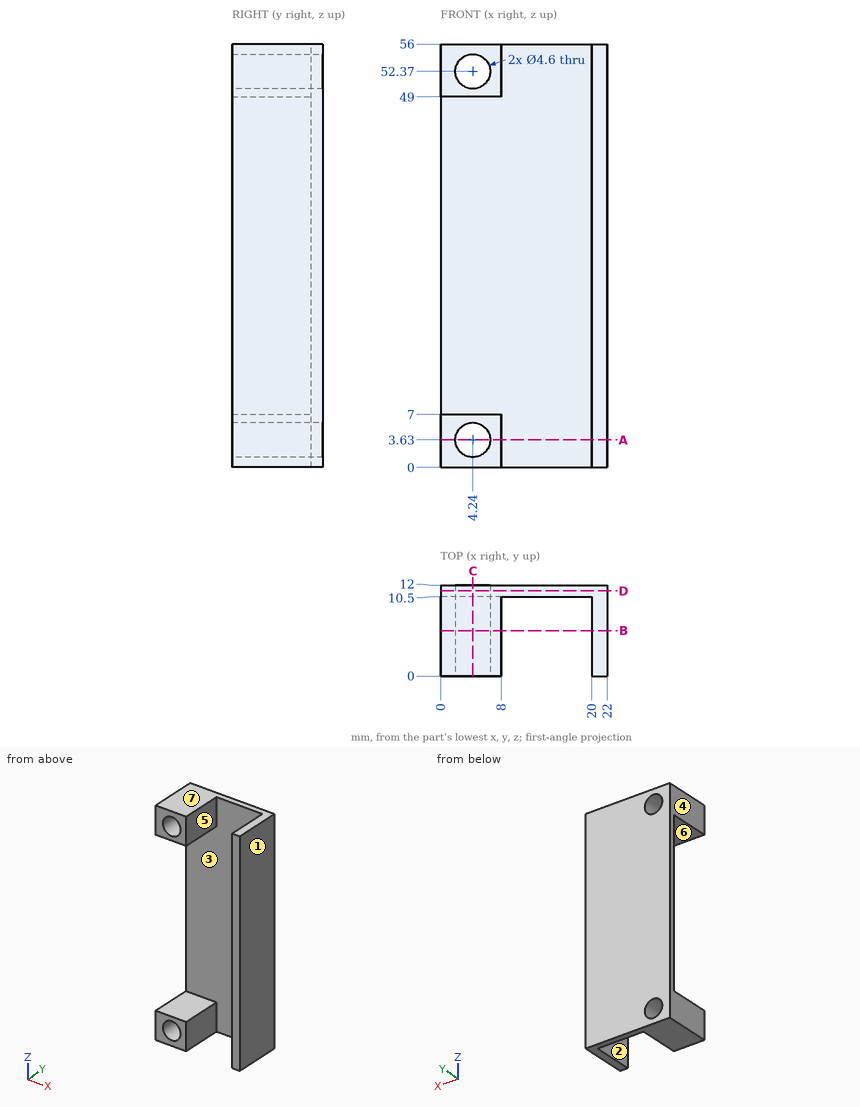
Geometry check sheet. Reference: drawing and pictorial views, mm from the part's lowest x, y, z. A direction names the side the tool comes from. Round coordinates to 2 decimals unless told otherwise and drop trailing zeros. Write each loop counter-clockwise with the first axis right and the second up, starting at its lowest first coordinate (ties: lowest second). Pieces come first, ordered by that corner, then holes. Notation, with made-up numbers: (19, -17) -> (47, -17) arc R25 cw to (47, -2) -> close; hole circle Ø5 at (23, 50.25). An arc over 180 degrees is marked (long way). Answer as CSV lines item,"result". Start each with the question number.
1) Section check C-C on x = 4.24. Enter the section's corners in (y, z), and give its area (3 significant figures).
2) Tool access check on the marked faces 5, 6 and 7. Record the directions out of +Z, -Z, +X, -X, +Y, -Y that give a thin tool (end or side, any length) a straight path to the whole face; none if there is none.
3) Section check D-D on y = 11.25. Enter the section's corners in (x, z), and give its area (3 significant figures).
4) Section check A-A on z = 3.63. Enter the section's corners in (x, y), and give its area (3 significant figures).
5) Section check B-B on y = 6. Enter the section's corners in (x, z), and give its area (3 significant figures).
6) Release check for a two-part mould opening along X. For the marked faces 1, 2, 3 and 4 record: pulls with the +X half, pulls with the -X half, needs draft (parallel to the pull), parting line crosses it, or undercut.
7) Material ranges on line 1 (X direction, y = 8.25, z = 52.37); line 2 (X direction, y = 7.5, z = 50); line 3 (Y direction, x = 17.75, z = 11), recorded low to high. Write a range as from..to.
8) Go/stop test with flat-tipped pins: P1, Ø3, axis at y = 4, z = 38, coming from the -X side; P2, Ø2, axis at x = 10.5, y = 5, coming from the -Z side (3 decimals); P3, Ø6, axis at x = 8, z = 38.5, coming from the -Y side; P4, Ø1.5, axis at x = 3.5, y = 4, coming from the -Z side. Record where each tip stops, or that it passes through.
Found:
1,outline,"(0, 0) -> (12, 0) -> (12, 1.33) -> (0, 1.33) -> close; (0, 5.93) -> (12, 5.93) -> (12, 50.07) -> (0, 50.07) -> (0, 49) -> (10.5, 49) -> (10.5, 7) -> (0, 7) -> close; (0, 54.67) -> (12, 54.67) -> (12, 56) -> (0, 56) -> close"
1,area,"121 mm^2"
2,face 5,"+Z, -Z, -Y"
2,face 6,"-X, -Y"
2,face 7,"+Z, +X, -X, +Y, -Y"
3,outline,"(0, 0) -> (22, 0) -> (22, 56) -> (0, 56) -> close; hole circle Ø4.6 at (4.24, 3.63); hole circle Ø4.6 at (4.24, 52.37)"
3,area,"1,200 mm^2"
4,outline,"(0, 0) -> (1.94, 0) -> (1.94, 12) -> (0, 12) -> close; (6.54, 0) -> (8, 0) -> (8, 10.5) -> (20, 10.5) -> (20, 0) -> (22, 0) -> (22, 12) -> (6.54, 12) -> close"
4,area,"82.8 mm^2"
5,outline,"(0, 0) -> (8, 0) -> (8, 7) -> (0, 7) -> close; (0, 49) -> (8, 49) -> (8, 56) -> (0, 56) -> close; (20, 0) -> (22, 0) -> (22, 56) -> (20, 56) -> close; hole circle Ø4.6 at (4.24, 3.63); hole circle Ø4.6 at (4.24, 52.37)"
5,area,"191 mm^2"
6,face 1,"pulls with the +X half"
6,face 2,"undercut"
6,face 3,"undercut"
6,face 4,"pulls with the -X half"
7,line 1,"x = 0..1.94, 6.54..8, 20..22"
7,line 2,"x = 0..8, 20..22"
7,line 3,"y = 10.5..12"
8,P1,"stops at x = 20"
8,P2,"passes through"
8,P3,"stops at y = 10.5"
8,P4,"stops at z = 0"
